Answer from the drawing. Dimensions are ordinates in mm from the lowest x, y and z of the part. A direction names the side the tool comes from. Give positions to 0.01 mm unless a question says otherwise; leave off trailing zeros. Write each loop counter-clockwise with the first axis right and the second up, starting at its lowest first coordinate (ties: lowest second). Pieces come first, ordered by that corner, then holes. Notation, with made-up numbers: (48, 89) -> (85, 89) arc R30 ccw to (85, 119) -> close; hole circle Ø10 at (21.25, -39.5). An arc over 180 degrees is marked (long way). Use a Markdown table: item, result. Add a question column.
Q1. Consider line 1 (X direction, y = 48.5, z = 13.5); line 2 (Y direction, x = 55, z = 20). Determine where each line is inside the solid, lowest interval first.
Q2. Section C-C, the plane x = 29.5 is taken. Give the vertices of the cut face in (y, z).
Q3. Each of these flat-tipped pins is pushed along its axis until it touches: pin 1 Ø13 at (y, z) = (31.5, 29) entering from -X; pin 2 Ø5 at (x, z) = (34, 10.5) entering from -Y. Where does it stop, or does it pass through?
Q4. Section A-A, the plane y = 23.5 is taken. Give the vertices of the cut face in (x, z), plus the area to 3 significant figures.
Q5. For a pull along Y with two mould halves and no side action, classify the marked faces 3, 4 and 5 as pulls with the +Y half, pulls with the -Y half, needs draft (parallel to the pull), parting line crosses it, or undercut.
Q6. For the marked faces 1 and 2, determine the directions among +Z, -Z, +X, -X, +Y, -Y from which every point of the face is accessible in a straight line to the end or side of a thin tool.
Q7. Section B-B, the plane z = 8 is taken. Give the vertices of the cut face in (x, y).
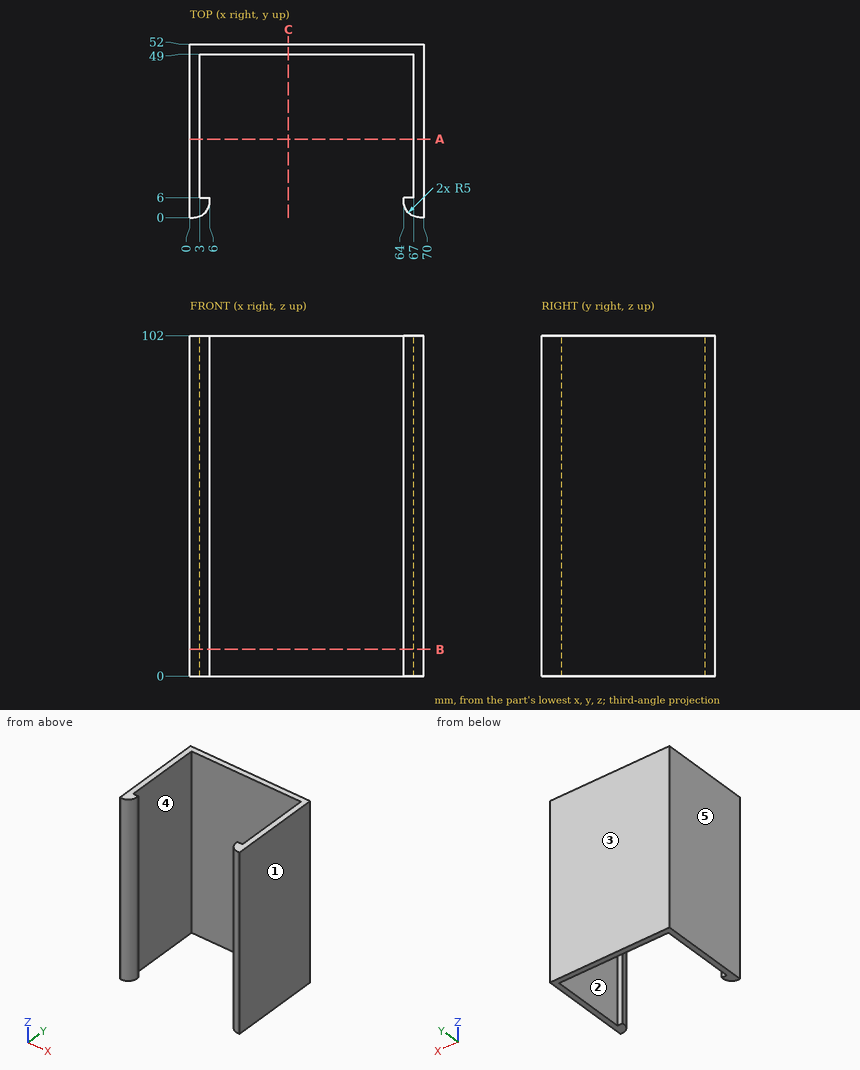
Result set:
| question | item | result |
|---|---|---|
| 1 | line 1 | x = 0 to 3, 67 to 70 |
| 1 | line 2 | y = 49 to 52 |
| 2 | outline | (49, 0) -> (52, 0) -> (52, 102) -> (49, 102) -> close |
| 3 | pin 1 | stops at x = 0 |
| 3 | pin 2 | stops at y = 49 |
| 4 | outline | (0, 0) -> (3, 0) -> (3, 102) -> (0, 102) -> close; (67, 0) -> (70, 0) -> (70, 102) -> (67, 102) -> close |
| 4 | area | 612 mm2 |
| 5 | face 3 | pulls with the +Y half |
| 5 | face 4 | undercut |
| 5 | face 5 | needs draft |
| 6 | face 1 | +Z, -Z, +X, +Y, -Y |
| 6 | face 2 | +Z, -Z |
| 7 | outline | (0, 0) -> (1, 0) arc R5 ccw to (6, 5) -> (6, 6) -> (3, 6) -> (3, 49) -> (67, 49) -> (67, 6) -> (64, 6) -> (64, 5) arc R5 ccw to (69, 0) -> (70, 0) -> (70, 52) -> (0, 52) -> close |
